from build123d import *

# Parameters (mm, degrees)
F0_R     = 4.5
F0_R_2   = 4
F1_DEPTH = 1.5875
F2_R     = 4
F3_DEPTH = 8.9
F4_R     = 4
F5_W     = 0.508
F5_H     = 0.508
F5_W_2   = 0.51
F5_H_2   = 0.51
F6_DEPTH = 5


with BuildPart() as f1:
    # F0 (on Front) → F1 (new body)
    with BuildSketch(Plane.XZ):
        Circle(F0_R)
        Circle(F0_R_2, mode=Mode.SUBTRACT)
        Circle(F0_R_2)
    extrude(amount=-F1_DEPTH)

    # F2 (on face) → F3 (join)
    with BuildSketch(Plane.XZ):
        Circle(F2_R)
    extrude(amount=F3_DEPTH)

    # F4
    f4_edges = [f1.edges().sort_by_distance(p)[0] for p in [
        (-4, -8.9, 0),
    ]]
    fillet(f4_edges, radius=F4_R)

    # F5 (on face) → F6 (join)
    with BuildSketch(Plane(origin=(0, 1.5875, 0), x_dir=(-1, 0, 0), z_dir=(0, 1, 0))):
        with Locations((0, 1.905)):
            Rectangle(F5_W, F5_H)
        with Locations((0, 0.635)):
            Rectangle(F5_W_2, F5_H_2)
        with Locations((0, -0.635)):
            Rectangle(F5_W_2, F5_H_2)
        with Locations((0, -1.905)):
            Rectangle(F5_W, F5_H)
    extrude(amount=F6_DEPTH)


solid = f1.part
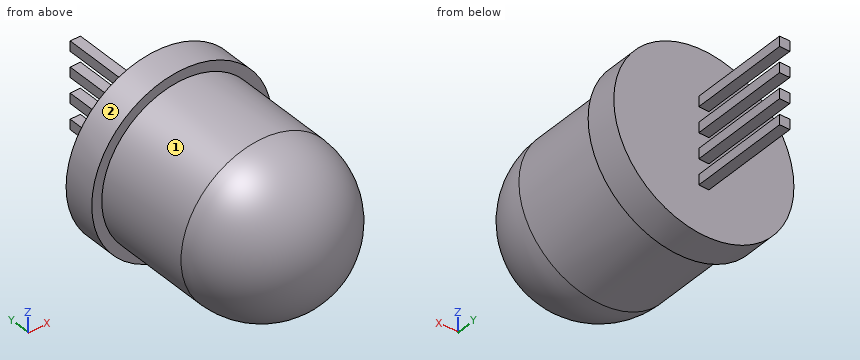
Read the model definition and answer for the solid it produces. Units are mm, in the model's axes. Face numbers are marked on the shaded views. A direction names the side the tool comes from. Round coordinates to 2 decimals unless told otherwise and drop trailing zeros. Loops run counter-clockwise (first coordinate to the right, second up) from the corner with the lowest first, then second, coordinate; pieces in that order, holes last. Notation, with made-up numbers: (26.5, -38.5) - (53.5, -38.5) arc R15 ccw to (53.5, -32.5) - close; hole circle Ø10 at (32, 40.25). An arc over 180 degrees is marked (long way). One line per question, with ' | ' between items. Start each with the question number.
Q1. Section B-B on z = 0 is taken. Give the vertices of the cut face in (x, y).
Q2. Section C-C on x = 0 is taken. Give the vertices of the cut face in (y, z).
Q3. Section D-D on y = 0.5 is taken. Give the vertices of the cut face in (x, z), plus the area to 3 significant figures.
Q4. Flat-ended cylindrical pins translate along their axes: pin 1 (0.6 mm diameter, centred on y = 4.5, z = 0.5, fed in from -X) (3 decimals); pin 2 (1.5 mm diameter, centred on x = -2.5, y = 3, fed in from +Z); pin 3 (1 mm diameter, centred on x = 1.5, y = 1, fed in from -Z); pin 4 (0.6 mm diameter, centred on x = 0, y = 3.5, fed in from +Z). Find the tip coordinate at first contact, or state that the pin passes through.
Q5. For the marked faces 1 and 2, determine the directions among +Z, -Z, +X, -X, +Y, -Y from which every point of the face is accessible in a straight line to the end or side of a thin tool.
Q6. Find the intervals of material crossed by L1, parallel to X at y = 5.25, z = 1.75; L2, parallel to Y at x = 4.25, z = -0.25; L3, parallel to X at y = -3, z = -1.5, in increasing order.
Q7. Section A-A on y = 2.5 is taken. Give the vertices of the cut face in (x, z) (3 decimals).
Established:
1) outline: (-4.5, 0) - (-4, 0) - (-4, -4.9) arc R4 ccw to (4, -4.9) - (4, 0) - (4.5, 0) - (4.5, 1.59) - (-4.5, 1.59) - close
2) outline: (-4.9, -4) - (0, -4) - (0, -4.5) - (1.59, -4.5) - (1.59, -2.16) - (6.59, -2.16) - (6.59, -1.65) - (1.59, -1.65) - (1.59, -0.89) - (6.59, -0.89) - (6.59, -0.38) - (1.59, -0.38) - (1.59, 0.38) - (6.59, 0.38) - (6.59, 0.89) - (1.59, 0.89) - (1.59, 1.65) - (6.59, 1.65) - (6.59, 2.16) - (1.59, 2.16) - (1.59, 4.5) - (0, 4.5) - (0, 4) - (-4.9, 4) arc R4 ccw to start
3) outline: circle Ø9 at (0, 0) | area: 63.6 mm²
4) pin 1: x = -0.255 | pin 2: through | pin 3: z = -4.39 | pin 4: z = 2.16
5) face 1: -Y | face 2: +Y, -Y
6) L1: -0.25 to 0.25 | L2: 0 to 1.59 | L3: -3.71 to 3.71
7) outline: (-0.255, -0.89) - (0.255, -0.89) - (0.255, -0.38) - (-0.255, -0.38) - close; (-0.255, 0.38) - (0.255, 0.38) - (0.255, 0.89) - (-0.255, 0.89) - close; (-0.254, -2.159) - (0.254, -2.159) - (0.254, -1.651) - (-0.254, -1.651) - close; (-0.254, 1.651) - (0.254, 1.651) - (0.254, 2.159) - (-0.254, 2.159) - close
